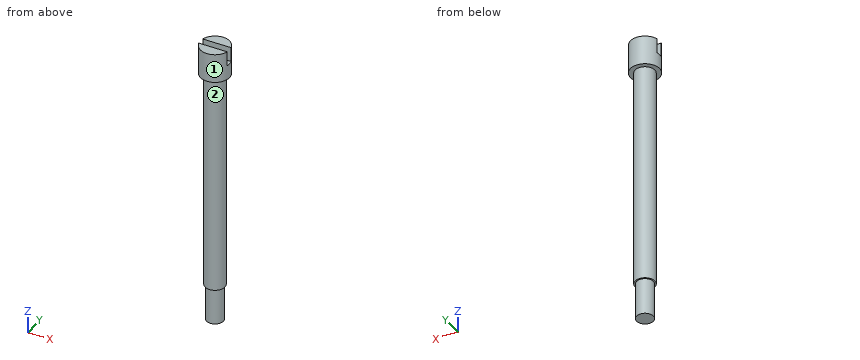
from build123d import *

# Parameters (mm, degrees)
SKETCH1_R           = 1.35
BOSS_EXTRUDE1_DEPTH = 35.5
SKETCH2_R           = 2
BOSS_EXTRUDE2_DEPTH = 4
SKETCH3_W           = 4
SKETCH3_H           = 1
CUT_EXTRUDE1_DEPTH  = 2
SKETCH4_OUTSIDE_W   = 13.98
SKETCH4_OUTSIDE_H   = 13.98
SKETCH4_OUTSIDE_R   = 1.15
CUT_EXTRUDE2_DEPTH  = 5


with BuildPart() as part:
    # Sketch1 → Boss-Extrude1 (new body)
    with BuildSketch(Plane.XY):
        Circle(SKETCH1_R)
    extrude(amount=BOSS_EXTRUDE1_DEPTH)

    # Sketch2 → Boss-Extrude2 (add)
    with BuildSketch(Plane.XY.offset(35.5)):
        Circle(SKETCH2_R)
    extrude(amount=BOSS_EXTRUDE2_DEPTH)

    # Sketch3 → Cut-Extrude1 (cut)
    with BuildSketch(Plane.XY.offset(39.5)):
        Rectangle(SKETCH3_W, SKETCH3_H)
    extrude(amount=-CUT_EXTRUDE1_DEPTH, mode=Mode.SUBTRACT)

    # Sketch4 outside → Cut-Extrude2 (cut)
    with BuildSketch(Plane(origin=(0, 0, 0), x_dir=(-1, 0, 0), z_dir=(0, 0, -1))):
        Rectangle(SKETCH4_OUTSIDE_W, SKETCH4_OUTSIDE_H)
        Circle(SKETCH4_OUTSIDE_R, mode=Mode.SUBTRACT)
    extrude(amount=-CUT_EXTRUDE2_DEPTH, mode=Mode.SUBTRACT)


solid = part.part
Read the model definition and answer for the solid it produces. Units are mm, in the model's axes. Face numbers are marked on the shaded views. A direction names the side the tool comes from. Give positions to 0.01 mm unless a question says otherwise; leave off trailing zeros. Write each loop counter-clockwise with the first axis right and the second up, starting at its lowest first coordinate (ties: lowest second). Pieces come first, ordered by that corner, then holes. Notation, with made-up numbers: (66.25, -13.75) -> (114.25, -13.75) arc R10 cw to (114.25, -1.75) -> close; hole circle Ø11 at (3.5, 31). An arc over 180 degrees is marked (long way). Answer as a JSON object with one key per item and string values. Group by question number.
1) Find section B-B (x = 0). Write down the section's boundary in (y, z).
2) Find section A-A (y = 0). Write down the section's boundary in (x, z).
3) A tool of negligible diameter and unlimited length cuts with its end or side. For the marked faces 1 and 2, from which of +Z, -Z, +X, -X, +Y, -Y can it reach the whole face along a straight path? Write none if from no direction.
4) Consider L1, parallel to Z at x = 0.55, y = 1.1; L2, parallel to Z at x = -1.15, y = 1.05; L3, parallel to X at y = -0.05, z = 20. Determine where each line is inside the solid, lowest interval first. Write a range as from..to.
5) Each of these flat-tipped pins is pushed along its axis until it touches: P1, Ø1.5, axis at y = 1, z = 32, coming from the +X side; P2, Ø2, axis at y = 0, z = 18, coming from the -X side; P3, Ø1, axis at x = -1, z = 38.5, coming from the +Y side; P4, Ø1.2, axis at x = 0, y = -1, coming from the -Z side. Where does it stop, or does it pass through?
6) Find section C-C (z = 9.5). Write down the section's boundary in (x, y), and give its area (3 significant figures).
Values follow:
{
 "1": {"outline": "(-2, 35.5) -> (-1.35, 35.5) -> (-1.35, 5) -> (-1.15, 5) -> (-1.15, 0) -> (1.15, 0) -> (1.15, 5) -> (1.35, 5) -> (1.35, 35.5) -> (2, 35.5) -> (2, 39.5) -> (0.5, 39.5) -> (0.5, 37.5) -> (-0.5, 37.5) -> (-0.5, 39.5) -> (-2, 39.5) -> close"},
 "2": {"outline": "(-2, 35.5) -> (-1.35, 35.5) -> (-1.35, 5) -> (-1.15, 5) -> (-1.15, 0) -> (1.15, 0) -> (1.15, 5) -> (1.35, 5) -> (1.35, 35.5) -> (2, 35.5) -> (2, 37.5) -> (-2, 37.5) -> close"},
 "3": {"face 1": "+Z, -Z", "face 2": "-Z"},
 "4": {"L1": "z = 5..39.5", "L2": "z = 35.5..39.5", "L3": "x = -1.35..1.35"},
 "5": {"P1": "stops at x = 1.33", "P2": "stops at x = -1.35", "P3": "stops at y = 1.94", "P4": "stops at z = 0"},
 "6": {"outline": "circle Ø2.7 at (0, 0)", "area": "5.73 mm2"}
}
